The listing builds one solid part. Answer for the finished solid, in the listing's coordinates (mm). Face numbers are marked on the shaded views. A direction names the side the tool comes from. Round coordinates to 2 decimals unless told otherwise and drop trailing zeros. Order: outer loops, then holes, each group sorted by start corner. A loop starts at its lowest first (then second) coordinate and runs counter-clockwise, first axis right, second up. Notation, with made-up numbers: (13.5, 62.5) -> (49.5, 62.5) arc R30 ccw to (49.5, 99.5) -> close; hole circle Ø3 at (7, -25). An arc over 180 degrees is marked (long way). Answer in a Markdown table with one row per item. Add a question column.
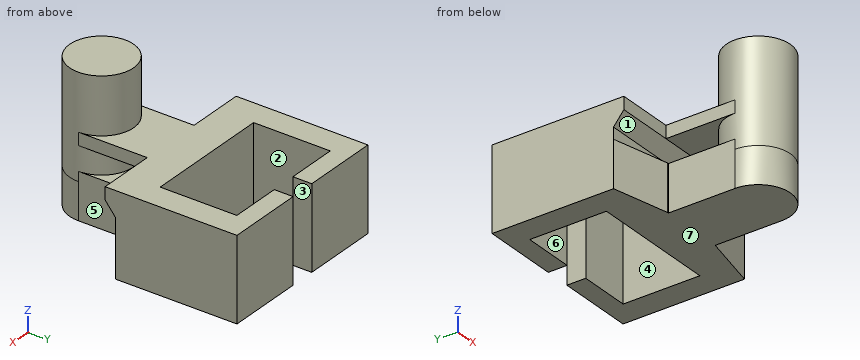
```python
from build123d import *

# Parameters (mm, degrees)
SKETCH1_R                = 15.875
BOSS_EXTRUDE1_DEPTH      = 50.8
SKETCH2_W                = 31.75
SKETCH2_H                = 50.8
BOSS_EXTRUDE2_DEPTH      = 4.7625
SKETCH3_W                = 88.9
SKETCH3_H                = 41.148
BOSS_EXTRUDE3_DEPTH      = 41.2496
CUT_EXTRUDE2_DEPTH       = 111.191148756
BOSS_EXTRUDE4_REACH      = 96.879
BOSS_EXTRUDE4_END_RADIUS = 15.875
SKETCH12_W               = 31.75
SKETCH12_H               = 6.203370687
SKETCH13_W               = 31.75
SKETCH13_H               = 4.7625
BOSS_EXTRUDE5_DEPTH      = 11.43
SKETCH14_W               = 38.1254
SKETCH14_H               = 41.148
BOSS_EXTRUDE6_DEPTH      = 7.62
SKETCH20_W               = 31.75
SKETCH20_H               = 5.130323172
BOSS_EXTRUDE7_DEPTH      = 6.35
CUT_EXTRUDE3_DEPTH       = 128.097501113
BOSS_EXTRUDE8_START      = 18.19275
BOSS_EXTRUDE8_DEPTH      = 18.19275
SKETCH25_W               = 28.575
SKETCH25_H               = 22.95525
BOSS_EXTRUDE10_DEPTH     = 6.35
CUT_EXTRUDE4_DEPTH       = 119.44527458
BOSS_EXTRUDE11_DEPTH     = 28.575
BOSS_EXTRUDE12_DEPTH     = 28.575


with BuildPart() as part:
    # Sketch1 → Boss-Extrude1 (new body)
    with BuildSketch(Plane.XY):
        Circle(SKETCH1_R)
    extrude(amount=BOSS_EXTRUDE1_DEPTH)

    # Sketch2 → Boss-Extrude2 (add)
    with BuildSketch(Plane(origin=(0, 0, 0), x_dir=(-1, 0, 0), z_dir=(0, 0, -1))):
        with Locations((0, 25.4)):
            Rectangle(SKETCH2_W, SKETCH2_H)
    extrude(amount=-BOSS_EXTRUDE2_DEPTH)

    # Sketch3 → Boss-Extrude3 (add)
    with BuildSketch(Plane(origin=(0, 50.8, 0), x_dir=(1, 0, 0), z_dir=(0, 1, 0))):
        with Locations((0, -2.38125)):
            Rectangle(SKETCH3_W, SKETCH3_H)
    extrude(amount=BOSS_EXTRUDE3_DEPTH)

    # Sketch5 → Cut-Extrude2 (cut, through all)
    with BuildSketch(Plane.XY.offset(22.95525)):
        Polygon((-6.3246, 92.0496), (-6.3246, 90.297), (-31.70428, 90.297), (-31.70428, 52.2224), (31.70428, 52.2224), (31.70428, 90.297), (6.3246, 90.297), (6.3246, 92.0496), align=None)
    extrude(amount=-CUT_EXTRUDE2_DEPTH, mode=Mode.SUBTRACT)

    # Boss-Extrude4: up to this cylinder (the profile starts outside it)
    boss_extrude4_end = Plane(origin=(0, 0, 19.853565), z_dir=(0, 0, -1)) * Cylinder(BOSS_EXTRUDE4_END_RADIUS, 226.508, mode=Mode.PRIVATE)
    # Sketch12 → Boss-Extrude4 (add, up to the surface)
    with BuildSketch(Plane.XZ.offset(-50.8), mode=Mode.PRIVATE) as boss_extrude4_sk1:
        with Locations((0, 19.853564657)):
            Rectangle(SKETCH12_W, SKETCH12_H)
    boss_extrude4_tool1 = extrude(boss_extrude4_sk1.sketch, amount=BOSS_EXTRUDE4_REACH, mode=Mode.PRIVATE) - boss_extrude4_end
    add(boss_extrude4_tool1.solids().sort_by_distance((0, 50.8, 19.853565))[0])

    # Sketch13 → Boss-Extrude5 (add)
    with BuildSketch(Plane.XZ.offset(-50.8)):
        Polygon((-44.45, 22.95525), (-15.875, 22.95525), (-15.875, 16.751879313), (15.875, 16.751879313), (15.875, 22.95525), (44.45, 22.95525), (44.45, -18.19275), (-44.45, -18.19275), align=None)
        with Locations((0, 2.38125)):
            Rectangle(SKETCH13_W, SKETCH13_H, mode=Mode.SUBTRACT)
    extrude(amount=BOSS_EXTRUDE5_DEPTH)

    # Sketch14 → Boss-Extrude6 (add)
    with BuildSketch(Plane(origin=(0, 92.0496, 0), x_dir=(1, 0, 0), z_dir=(0, 1, 0))):
        with Locations((-25.3873, -2.38125)):
            Rectangle(SKETCH14_W, SKETCH14_H)
        with Locations((25.3873, -2.38125)):
            Rectangle(SKETCH14_W, SKETCH14_H)
    extrude(amount=BOSS_EXTRUDE6_DEPTH)

    # Sketch20 → Boss-Extrude7 (add)
    with BuildSketch(Plane(origin=(0, 0, 16.751879313), x_dir=(-1, 0, 0), z_dir=(0, 0, -1))):
        with Locations((0, 36.804838414)):
            Rectangle(SKETCH20_W, SKETCH20_H)
    extrude(amount=BOSS_EXTRUDE7_DEPTH)

    # Sketch21 → Cut-Extrude3 (cut, through all)
    with BuildSketch(Plane(origin=(15.875, 0, 0), x_dir=(0, 0, -1), z_dir=(1, 0, 0))):
        Polygon((-16.751879313, 34.239676828), (-10.401879313, 39.37), (-10.401879313, 34.239676828), align=None)
    extrude(amount=-CUT_EXTRUDE3_DEPTH, mode=Mode.SUBTRACT)

    # Sketch22 → Boss-Extrude8 (add)
    with BuildSketch(Plane(origin=(0, 0, 0), x_dir=(-1, 0, 0), z_dir=(0, 0, -1)).offset(BOSS_EXTRUDE8_START)):
        with BuildLine():
            Line((-15.875, 39.37), (15.875, 39.37))
            Line((15.875, 39.37), (15.875, 0))
            ThreePointArc((15.875, 0), (0, -15.875), (-15.875, 0))
            Line((-15.875, 0), (-15.875, 39.37))
        make_face()
    extrude(amount=-BOSS_EXTRUDE8_DEPTH)

    # Sketch25 → Boss-Extrude10 (add)
    with BuildSketch(Plane.XZ.offset(-39.37)):
        with Locations((-30.1625, -6.715125)):
            Rectangle(SKETCH25_W, SKETCH25_H)
        with Locations((30.1625, -6.715125)):
            Rectangle(SKETCH25_W, SKETCH25_H)
    extrude(amount=BOSS_EXTRUDE10_DEPTH)

    # Sketch26 → Cut-Extrude4 (cut, through all)
    with BuildSketch(Plane.XY.offset(4.7625)):
        Polygon((-44.45, 39.37), (-16.350375035, 33.02), (-44.45, 33.02), align=None)
        Polygon((15.875, 33.02), (44.45, 39.37), (44.45, 33.02), align=None)
    extrude(amount=-CUT_EXTRUDE4_DEPTH, mode=Mode.SUBTRACT)

    # Sketch27 → Boss-Extrude11 (add)
    with BuildSketch(Plane.ZY.offset(15.875)):
        Polygon((16.751879313, 34.239676828), (22.95525, 34.239676828), (22.95525, 39.37), (10.401879313, 39.37), align=None)
    extrude(amount=BOSS_EXTRUDE11_DEPTH)

    # Sketch28 → Boss-Extrude12 (add)
    with BuildSketch(Plane(origin=(15.875, 0, 0), x_dir=(0, 0, -1), z_dir=(1, 0, 0))):
        Polygon((-16.751879313, 34.239676828), (-22.95525, 34.239676828), (-22.95525, 39.37), (-10.401879313, 39.37), align=None)
    extrude(amount=BOSS_EXTRUDE12_DEPTH)


solid = part.part
```
1. Each of these flat-tipped pins is pushed along its axis until it touches: pin 1 (3 mm diameter, centred on x = 21, z = 6.5, fed in from -Y); pin 2 (6 mm diameter, centred on x = 9.5, y = 30, fed in from +Z); pin 3 (10 mm diameter, centred on x = -21, z = 7.5, fed in from -Y); pin 4 (3 mm diameter, centred on x = 17.5, z = 24.5, fed in from +Y). Where does it stop, or does it pass through?
2. The part is cut by section A-A (x = 0). Give the vertices of the cut face in (y, z) (1 decimal).
3. Straight lines are drawn through the part: line 1 along X through (y, z) = (58, -10.5); line 2 along Z through (x, y) = (35.5, 54); line 3 along Y through (x, z) = (38.5, 9). For each, find the intervals that lie inside material, in ascending order.
4. The part is cut by section B-B (y = 79.5). Give the vertices of the cut face in (x, z), then the cut area to 3 significant figures.
5. For the marked faces 1, 2 and 3, determine the directions among +Z, -Z, +X, -X, +Y, -Y from which every point of the face is accessible in a straight line to the end or side of a thin tool.
6. The part is cut by section C-C (z = -11). Give the vertices of the cut face in (x, y) (3 decimals).
7. The mould has two halves that part along X. Classify the marked faces 4, 5, 6 and 7: released by +X, released by -X, zero draft, split by the parting line, or undercut.
8. The part is cut by section D-D (x = 24). Give the vertices of the cut face in (y, z).
Report:
| question | item | result |
|---|---|---|
| 1 | pin 1 | stops at y = 39.37 |
| 1 | pin 2 | stops at z = 22.96 |
| 1 | pin 3 | stops at y = 33.13 |
| 1 | pin 4 | passes through |
| 2 | outline | (-15.9, -18.2) -> (52.2, -18.2) -> (52.2, 23) -> (15.9, 23) -> (15.9, 50.8) -> (-15.9, 50.8) -> close; hole (15.9, 4.8) -> (39.4, 4.8) -> (39.4, 10.4) -> (34.2, 16.8) -> (15.9, 16.8) -> close |
| 3 | line 1 | x = -44.45 to -31.7, 31.7 to 44.45 |
| 3 | line 2 | z = -18.19 to 22.96 |
| 3 | line 3 | y = 39.37 to 99.67 |
| 4 | outline | (-44.45, -18.19) -> (-31.7, -18.19) -> (-31.7, 22.96) -> (-44.45, 22.96) -> close; (31.7, -18.19) -> (44.45, -18.19) -> (44.45, 22.96) -> (31.7, 22.96) -> close |
| 4 | area | 1,050 mm^2 |
| 5 | face 1 | +X, -X |
| 5 | face 2 | +Z, -Z |
| 5 | face 3 | +Z, -Z, +Y |
| 6 | outline | (-44.45, 39.37) -> (-16.35, 33.02) -> (-15.875, 33.02) -> (-15.875, 0) arc R15.875 ccw to (15.875, 0) -> (15.875, 33.02) -> (44.45, 39.37) -> (44.45, 99.67) -> (6.325, 99.67) -> (6.325, 90.297) -> (31.704, 90.297) -> (31.704, 52.222) -> (-31.704, 52.222) -> (-31.704, 90.297) -> (-6.325, 90.297) -> (-6.325, 99.67) -> (-44.45, 99.67) -> close |
| 7 | face 4 | undercut |
| 7 | face 5 | released by +X |
| 7 | face 6 | undercut |
| 7 | face 7 | zero draft |
| 8 | outline | (34.24, 16.75) -> (39.37, 10.4) -> (39.37, 4.76) -> (34.83, 4.76) -> (34.83, -18.19) -> (52.22, -18.19) -> (52.22, 22.96) -> (34.24, 22.96) -> close; (90.3, -18.19) -> (99.67, -18.19) -> (99.67, 22.96) -> (90.3, 22.96) -> close |
